Part print with two shaded views. Sizes in mm from the minimum x, y, z corner. A direction names the side the tool comes from. Round coordinates to 2 decimals unless told otherwise and drop trailing zeros. Order: outer loops, then holes, each group sorted by start corner. A loop starts at its lowest first (then second) coordinate and runs counter-clockwise, first axis right, second up. Notation, with made-up numbers: (48.5, 73) - (93.5, 73) arc R36 ccw to (93.5, 110) - close; hole circle Ø9 at (46, -17.75). An arc over 180 degrees is marked (long way). Answer as CSV lines item,"result". Start each with the question number.
1. Band-saw the part on A-A on z = 14. List the corners of the cut face in (x, y) (1 decimal), then the cut area to 3 significant figures.
2. Wall check: line 1 along Y through (x, z) = (12.7, 2.2) (1 decimal); line 2 along X through (y, z) = (12.75, 11) (1 decimal); line 3 along Z through (x, y) = (21, 21.5). Give the ranges that are in metal, low to high. Write a range as [from, to].
3. Pin check, flat tips, straight feed: pin 1 Ø2 at (x, z) = (14.5, 13) entering from +Y (1 decimal); pin 2 Ø1 at (y, z) = (19, 12.5) entering from +X (1 decimal); pin 3 Ø3 at (x, z) = (12.5, 13) entering from -Y. Stop position of each tip, or through.
4. Pull direction Z, two halves, no side cores. Call the marked faces 1, 2, 3 and 4: released by +Z, released by -Z, zero draft, split by the parting line, or undercut.
5. Band-saw the part on C-C on z = 10. List the corners of the cut face in (x, y) (1 decimal).
6. 3-axis set-ups, long thin cutter, end or side, ignore diameter. For the marked faces 5 and 6: which of +Z, -Z, +X, -X, +Y, -Y reach the whole face in a straight line?
7. Band-saw the part on B-B on x = 12.7. List the corners of the cut face in (y, z) (1 decimal).
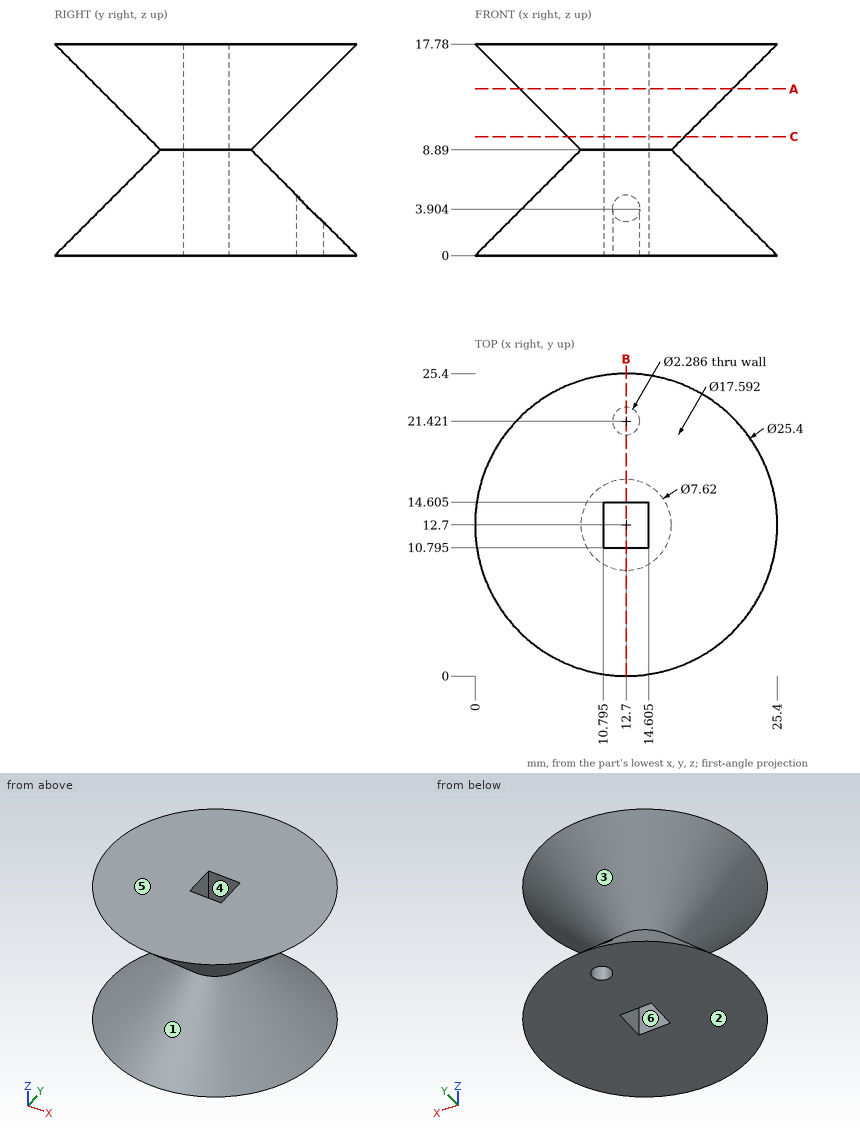
Reply:
1,outline,"circle Ø17.8 at (12.7, 12.7); hole (10.8, 10.8) - (14.6, 10.8) - (14.6, 14.6) - (10.8, 14.6) - close"
1,area,"235 mm2"
2,line 1,"y = [2.2, 10.8], [14.6, 20.3], [22.6, 23.2]"
2,line 2,"x = [6.8, 10.8], [14.6, 18.6]"
2,line 3,"z = [0, 0.6], [17.18, 17.78]"
3,pin 1,"stops at y = 21.5"
3,pin 2,"stops at x = 17.7"
3,pin 3,"stops at y = 3.28"
4,face 1,"undercut"
4,face 2,"released by -Z"
4,face 3,"undercut"
4,face 4,"zero draft"
5,outline,"circle Ø9.8 at (12.7, 12.7); hole (10.8, 10.8) - (14.6, 10.8) - (14.6, 14.6) - (10.8, 14.6) - close"
6,face 5,"+Z, +X, -X, +Y, -Y"
6,face 6,"+Z, -Z"
7,outline,"(0, 0) - (10.8, 0) - (10.8, 17.8) - (0, 17.8) - (8.9, 8.9) - close; (14.6, 0) - (20.3, 0) - (20.3, 5.1) - (16.5, 8.9) - (25.4, 17.8) - (14.6, 17.8) - close; (22.6, 0) - (25.4, 0) - (22.6, 2.8) - close"
